Design review of the part built by this model. Coordinates are the model's own, in mm. A direction names the side the tool comes from. Round coordinates to 2 decimals unless told otherwise and drop trailing zeros. Write each loop counter-clockwise with the first axis right and the second up, starting at its lowest first coordinate (ties: lowest second). Pieces come first, ordered by that corner, then holes. Notation, with made-up numbers: (1, 54) -> (5, 54) arc R15 cw to (5, 59) -> close; hole circle Ø3 at (-26, 76). An arc over 180 degrees is marked (long way). One line per question, with ' | ' between items. Start each with the question number.
1) Consider section A-A (y = 5.5). Give the boundary of the cut face in (x, z).
2) For faces 5 (the conical face through (0.095, -19.334, 0.365)), 6 (the conical face through (10.819, -38.246, 9.858)), 7 (the cylindrical face through (-0.16, -22.2, 7.53)), list the 3-axis set-ups (+Z, -Z, +X, -X, +Y, -Y) from which the entire face can be reached by the end or side of a thin tool; tool diameter is ignored.
3) Mouldability with a two-part tool opening along Y and no side actions: class faces 1 (the flat face through (-7.2, 0, 8)), 2 (the flat face through (-5, 0, 5)), 3 (the flat face through (-8, 1, 10)), 4 (the conical face through (10.819, -38.246, 0.142)) as +Y half, -Y half, draft (parallel to the pull), parting line (faces both ways), or undercut.
4) Consider section B-B (x = 0). Count the separate pieces of the cut face and the enclosed holes in it, then the cut area to 3 significant figures.
5) For probe 1 along Y at (x, z) = (0, 3.25); probe 2 along Y at (x, z) = (0, 7.75); probe 3 along X at (y, z) = (-8, 8.5), list the stretches that pass through material, from the lowest coordinate up.
6) Insertion check: pin 1 Ø6 at (x, y) = (4, 2.5) entering from +Z; pin 2 Ø10.5 at (x, y) = (1, 6) entering from +Z; pin 3 Ø5 at (x, y) = (5, -3.5) entering from +Z; pin 4 Ø6.5 at (x, y) = (0, -32) entering from -Z. Each pin has a flat end and moves straight along its axis. Give the tip position at first contact, or say it passes through.
7) Consider section C-C (y = -32). Give the boundary of the cut face in (x, z), then the cut area to 3 significant figures.
```python
from build123d import *

# Parameters (mm, degrees)
F0_W     = 25
F0_H     = 80
F0_R     = 3.5
F1_DEPTH = 10
F3_DEPTH = 5
F4_R     = 5
F5_SIZE  = 0.5
F6_R     = 0.5


with BuildPart() as f1:
    # F0 (on Top) → F1 (new body)
    with BuildSketch(Plane.XY):
        Rectangle(F0_W, F0_H)
        with Locations((0, -32)):
            Circle(F0_R, mode=Mode.SUBTRACT)
        with BuildLine():
            ThreePointArc((-4.2, 15), (0, 19.2), (4.2, 15))
            Line((4.2, 15), (4.2, -15))
            ThreePointArc((4.2, -15), (0, -19.2), (-4.2, -15))
            Line((-4.2, -15), (-4.2, 15))
        make_face(mode=Mode.SUBTRACT)
    extrude(amount=F1_DEPTH)

    # F2 (on face) → F3 (cut)
    with BuildSketch(Plane.XY.offset(10)):
        with BuildLine():
            Line((7.2, -15), (7.2, 15))
            ThreePointArc((7.2, 15), (0, 22.2), (-7.2, 15))
            Line((-7.2, 15), (-7.2, -15))
            ThreePointArc((-7.2, -15), (0, -22.2), (7.2, -15))
        make_face()
        with BuildLine():
            ThreePointArc((-4.2, 15), (0, 19.2), (4.2, 15))
            Line((4.2, 15), (4.2, -15))
            ThreePointArc((4.2, -15), (0, -19.2), (-4.2, -15))
            Line((-4.2, -15), (-4.2, 15))
        make_face(mode=Mode.SUBTRACT)
    extrude(amount=-F3_DEPTH, mode=Mode.SUBTRACT)

    # F4
    f4_edges = [f1.edges().sort_by_distance(p)[0] for p in [
        (12.5, 40, 5),
        (-12.5, -40, 5),
        (12.5, -40, 5),
        (-12.5, 40, 5),
    ]]
    fillet(f4_edges, radius=F4_R)

    # F5
    f5_edges = [f1.edges().sort_by_distance(p)[0] for p in [
        (0, 40, 10),
        (11.035534, 38.535534, 10),
        (-11.035534, 38.535534, 10),
        (12.5, 0, 10),
        (-12.5, 0, 10),
        (11.035534, -38.535534, 10),
        (-11.035534, -38.535534, 10),
        (0, -40, 10),
        (-3.5, -32, 10),
        (0, -22.2, 10),
        (7.2, 0, 10),
        (0, 22.2, 10),
        (-7.2, 0, 10),
        (0, 40, 0),
        (11.035534, 38.535534, 0),
        (-11.035534, 38.535534, 0),
        (12.5, 0, 0),
        (-12.5, 0, 0),
        (11.035534, -38.535534, 0),
        (-11.035534, -38.535534, 0),
        (0, -40, 0),
        (-3.5, -32, 0),
        (0, -19.2, 0),
        (-4.2, 0, 0),
        (0, 19.2, 0),
        (4.2, 0, 0),
    ]]
    chamfer(f5_edges, length=F5_SIZE)

    # F6
    f6_edges = [f1.edges().sort_by_distance(p)[0] for p in [
        (0, 22.2, 5),
    ]]
    fillet(f6_edges, radius=F6_R)


solid = f1.part
```
From the geometry:
1) outline: (-12.5, 0.5) -> (-12, 0) -> (-4.7, 0) -> (-4.2, 0.5) -> (-4.2, 5) -> (-6.7, 5) arc R0.5 cw to (-7.2, 5.5) -> (-7.2, 9.5) -> (-7.7, 10) -> (-12, 10) -> (-12.5, 9.5) -> close; (4.2, 0.5) -> (4.7, 0) -> (12, 0) -> (12.5, 0.5) -> (12.5, 9.5) -> (12, 10) -> (7.7, 10) -> (7.2, 9.5) -> (7.2, 5.5) arc R0.5 cw to (6.7, 5) -> (4.2, 5) -> close
2) face 5: -Z | face 6: +Z, +X, -Y | face 7: +Z
3) face 1: undercut | face 2: undercut | face 3: draft | face 4: -Y half
4) separate pieces: 3 | enclosed holes: 0 | area: 315 mm2
5) probe 1: y = -40 to -35.5, -28.5 to -19.2, 19.2 to 40 | probe 2: y = -40 to -35.5, -28.5 to -22.2, 22.2 to 40 | probe 3: x = -12.5 to -7.2, 7.2 to 12.5
6) pin 1: stops at z = 5.1 | pin 2: stops at z = 5 | pin 3: stops at z = 9.8 | pin 4: passes through
7) outline: (-12.5, 0.5) -> (-12, 0) -> (-4, 0) -> (-3.5, 0.5) -> (-3.5, 9.5) -> (-4, 10) -> (-12, 10) -> (-12.5, 9.5) -> close; (3.5, 0.5) -> (4, 0) -> (12, 0) -> (12.5, 0.5) -> (12.5, 9.5) -> (12, 10) -> (4, 10) -> (3.5, 9.5) -> close | area: 179 mm2
